Autodesk Inventor part; units mm, degrees
ref_plane "YZ Plane" through (0, 0, 0) normal (1, 0, 0) x (0, 1, 0)
ref_plane "XZ Plane" through (0, 0, 0) normal (0, 1, 0) x (-1, 0, 0)
ref_plane "XY Plane" through (0, 0, 0) normal (0, 0, 1) x (1, 0, 0)
sketch "Sketch1" plane through (0, 0, 0) normal (0, 1, 0) x (-1, 0, 0)
  line L0 (0, 0) -> (-57.15, 0)
  line L1 (-57.15, 0) -> (-57.15, -57.15)
  line L2 (-57.15, -57.15) -> (0, -57.15)
  line L3 (0, -57.15) -> (0, 0)
  circle A0 centre (-3.81, -3.81) radius 1.27
  line L4 (-28.575, 0) -> (-28.575, -57.15) construction
  line L5 (0, -28.575) -> (-57.15, -28.575) construction
  circle A1 centre (-3.81, -53.34) radius 1.27
  circle A2 centre (-53.34, -3.81) radius 1.27
  circle A3 centre (-53.34, -53.34) radius 1.27
  dimension "d0" = 57.15
  dimension "d1" = 57.15
  dimension "d2" = 3.81
  dimension "d3" = 2.54
  dimension "d4" = 3.81
extrude "Extrusion1" add sketch "Sketch1" along normal blind 1.6
sketch "Sketch2" plane through (0, 1.6, 0) normal (0, 1, 0) x (1, 0, 0)
  circle A0 centre (53.34, 53.34) radius 1.27
  circle A1 centre (53.34, 3.81) radius 1.27
  circle A2 centre (3.81, 53.34) radius 1.27
  circle A3 centre (3.81, 3.81) radius 1.27
  line L0 (0, 0) -> (57.15, 0)
  line L1 (57.15, 0) -> (57.15, 57.15)
  line L2 (57.15, 57.15) -> (0, 57.15)
  line L3 (0, 57.15) -> (0, 0)
  dimension "d7" = 49.53
properties part number "SFE PCB"
CAD build for the part. Positions are in the model's coordinates, mm. Round coordinates to 2 decimals unless told otherwise and drop trailing zeros. Order: outer loops, then holes, each group sorted by start corner. A loop starts at its lowest first (then second) coordinate and runs counter-clockwise, first axis right, second up. Notation, with made-up numbers: (3, 19) - (62, 19) arc R14 cw to (62, 39) - close; hole circle Ø5 at (70, 11). An arc over 180 degrees is marked (long way). Answer in a Markdown table with one row per item. Add a question column.
(1) Band-saw the part on A-A on z = -53.34. List the corners of the cut face in (x, y), and give its area (3 significant figures).
(2) Probe L1, parallel to Z at x = 53.34, y = 0.95; L2, parallel to X at y = 1.45, z = -4; L3, parallel to X at y = 0.1, z = -54.5. List the from-to ranges inside material, lowest first. Write a range as [from, to].
(3) Mould opens along X. For faces 1 (the face through (57.15, 1, -28)), 2 (the face through (29, 1.6, -28)), 3 (the face through (4.09, 0.79, -52.1)) say: +X half, -X half, draft (parallel to the pull), parting line (faces both ways), or undercut.
(4) Drop a flat-ended pin along its axis: pin 1 Ø1.5 at (x, z) = (53.34, -3.81) entering from -Y. Give the stop position or say it passes through.
(5) Band-saw the part on B-B on x = 53.34. List the corners of the cut face in (y, z), and give its area (3 significant figures).
Data:
| question | item | result |
|---|---|---|
| 1 | outline | (0, 0) - (2.54, 0) - (2.54, 1.6) - (0, 1.6) - close; (5.08, 0) - (52.07, 0) - (52.07, 1.6) - (5.08, 1.6) - close; (54.61, 0) - (57.15, 0) - (57.15, 1.6) - (54.61, 1.6) - close |
| 1 | area | 83.3 mm^2 |
| 2 | L1 | z = [-57.15, -54.61], [-52.07, -5.08], [-2.54, 0] |
| 2 | L2 | x = [0, 2.55], [5.07, 52.08], [54.6, 57.15] |
| 2 | L3 | x = [0, 3.29], [4.33, 52.82], [53.86, 57.15] |
| 3 | face 1 | +X half |
| 3 | face 2 | draft |
| 3 | face 3 | undercut |
| 4 | pin 1 | passes through |
| 5 | outline | (0, -57.15) - (1.6, -57.15) - (1.6, -54.61) - (0, -54.61) - close; (0, -52.07) - (1.6, -52.07) - (1.6, -5.08) - (0, -5.08) - close; (0, -2.54) - (1.6, -2.54) - (1.6, 0) - (0, 0) - close |
| 5 | area | 83.3 mm^2 |
